```python
from build123d import *

# Parameters (mm, degrees)
SKETCH014_W   = 8.5
SKETCH014_H   = 44
PAD_DEPTH     = 20
SKETCH008_R   = 1.5
HOLE_DEPTH    = 4
SKETCH018_R   = 1.5
HOLE002_DEPTH = 4


with BuildPart() as part:
    # Sketch014 → Pad (new body)
    with BuildSketch(Plane.XY):
        with Locations((-4.25, 22)):
            Rectangle(SKETCH014_W, SKETCH014_H)
    extrude(amount=PAD_DEPTH)

    # Sketch008 → Hole (cut)
    with BuildSketch(Plane.XY):
        with Locations((-4.250802, 4.5)):
            Circle(SKETCH008_R)
        with Locations((-4.25, 39.499999)):
            Circle(SKETCH008_R)
        with Locations((-4.254534, 22)):
            Circle(SKETCH008_R)
        with Locations((-4.25, 4.5)):
            Circle(SKETCH008_R)
    extrude(amount=HOLE_DEPTH, mode=Mode.SUBTRACT)

    # Sketch018 (on Face5 of Hole) → Hole002 (cut)
    with BuildSketch(Plane.XY.offset(20)):
        with Locations((-4.250802, 4.5)):
            Circle(SKETCH018_R)
        with Locations((-4.25, 39.499999)):
            Circle(SKETCH018_R)
        with Locations((-4.254534, 22)):
            Circle(SKETCH018_R)
        with Locations((-4.25, 4.5)):
            Circle(SKETCH018_R)
    extrude(amount=-HOLE002_DEPTH, mode=Mode.SUBTRACT)


solid = part.part
```
Build history of the part. All positions in model axes, mm. A direction names the side the tool comes from. Coordinates: 2 decimals unless noted, no trailing zeros. Order: outer loops, then holes, each group sorted by start corner. A loop starts at its lowest first (then second) coordinate and runs counter-clockwise, first axis right, second up. Notation, with made-up numbers: (30.5, 50) -> (77.5, 50) arc R19 cw to (77.5, 78) -> close; hole circle Ø3 at (27, -31.5). An arc over 180 degrees is marked (long way). Answer in a Markdown table with one row per item. Add a question column.
Q1. Drop a flat-ended pin along its axis: pin 1 (1.5 mm diameter, centred on x = -4, y = 5, fed in from -Z). Give the stop position or say it passes through.
Q2. Band-saw the part on A-A, the plane y = 4.5. List the corners of the cut face in (x, z), then the cut area to 3 significant figures.
Q3. Mould opens along X. For faces 4 (the face through (-8.5, 22, 10)), 5 (the face through (-4, 0, 10)), 6 (the face through (-4, 40, 4)), 7 (the face through (-4.445, 40.987, 18.028)) say: +X half, -X half, draft (parallel to the pull), parting line (faces both ways), or undercut.
Q4. Which spindle directions (+Z, -Z, +X, -X, +Y, -Y) get a long thin tool onto all of the face, cutting with end or side? Do faces 1 (the face through (0, 22, 10)), 2 (the face through (-4, 22, 16)), 3 (the face through (-4.445, 40.987, 1.972)). Say none if no direction does.
Q5. Wall check: line 1 along Y through (x, z) = (-4.25, 2.25); line 2 along X through (y, z) = (39.5, 17.2); line 3 along Y through (x, z) = (-5, 18.25). Give the ranges that are in metal, low to high. Write a range as [from, to].
Q6. Band-saw the part on B-B, the plane x = -3.5. List the corners of the cut face in (y, z).
Answers follow:
| question | item | result |
|---|---|---|
| 1 | pin 1 | z = 4 |
| 2 | outline | (-8.5, 0) -> (-5.75, 0) -> (-5.75, 4) -> (-2.75, 4) -> (-2.75, 0) -> (0, 0) -> (0, 20) -> (-2.75, 20) -> (-2.75, 16) -> (-5.75, 16) -> (-5.75, 20) -> (-8.5, 20) -> close |
| 2 | area | 146 mm^2 |
| 3 | face 4 | -X half |
| 3 | face 5 | draft |
| 3 | face 6 | undercut |
| 3 | face 7 | undercut |
| 4 | face 1 | +Z, -Z, +X, +Y, -Y |
| 4 | face 2 | +Z |
| 4 | face 3 | -Z |
| 5 | line 1 | [0, 3], [6, 20.5], [23.5, 38], [41, 44] |
| 5 | line 2 | [-8.5, -5.75], [-2.75, 0] |
| 5 | line 3 | [0, 3.2], [5.8, 20.7], [23.3, 38.2], [40.8, 44] |
| 6 | outline | (0, 0) -> (3.2, 0) -> (3.2, 4) -> (5.8, 4) -> (5.8, 0) -> (20.7, 0) -> (20.7, 4) -> (23.3, 4) -> (23.3, 0) -> (38.2, 0) -> (38.2, 4) -> (40.8, 4) -> (40.8, 0) -> (44, 0) -> (44, 20) -> (40.8, 20) -> (40.8, 16) -> (38.2, 16) -> (38.2, 20) -> (23.3, 20) -> (23.3, 16) -> (20.7, 16) -> (20.7, 20) -> (5.8, 20) -> (5.8, 16) -> (3.2, 16) -> (3.2, 20) -> (0, 20) -> close |
